```python
from build123d import *

# Parameters (mm, degrees)
F1_DEPTH = 5


with BuildPart() as f1:
    # F0 (on Top) → F1 (new body)
    with BuildSketch(Plane.XY):
        with BuildLine():
            ThreePointArc((3.1956666573, -6.9824714928), (2.7675285072, -8.5803048214), (1.5978333287, -9.75))
            Line((1.5978333287, -9.75), (4.793499986, -9.75))
            ThreePointArc((4.793499986, -9.75), (4.3653618359, -8.1521666713), (3.1956666573, -6.9824714928))
        make_face()
        with BuildLine():
            Line((-4.793499986, -9.75), (-1.5978333286, -9.75))
            ThreePointArc((-1.5978333286, -9.75), (-2.7675285072, -8.5803048214), (-3.1956666573, -6.9824714928))
            ThreePointArc((-3.1956666573, -6.9824714928), (-4.3653618359, -8.1521666713), (-4.793499986, -9.75))
        make_face()
        with BuildLine():
            ThreePointArc((3.1956666573, -6.9824714928), (4.3653618359, -8.1521666713), (4.793499986, -9.75))
            Line((4.793499986, -9.75), (12.3826613305, -9.75))
            Line((12.3826613305, -9.75), (17.9021666714, -9.75))
            ThreePointArc((17.9021666714, -9.75), (13.2777422874, 2.8582215277), (1.5978333286, 9.4863643814))
            Line((1.5978333286, 9.4863643814), (1.5978333287, -4.2149429855))
            ThreePointArc((1.5978333286, -4.2149429855), (2.7675285072, -5.3846381641), (3.1956666573, -6.9824714928))
        make_face()
        with BuildLine():
            Line((-17.9021666713, -9.75), (-4.793499986, -9.75))
            ThreePointArc((-4.793499986, -9.75), (-4.3653618359, -8.1521666713), (-3.1956666573, -6.9824714928))
            ThreePointArc((-3.1956666573, -6.9824714928), (-2.7675285072, -5.3846381641), (-1.5978333287, -4.2149429855))
            Line((-1.5978333286, -4.2149429855), (-1.5978333287, 9.4863643814))
            ThreePointArc((-1.5978333287, 9.4863643814), (-13.2777422874, 2.8582215277), (-17.9021666713, -9.75))
        make_face()
        with BuildLine():
            ThreePointArc((-1.5978333287, -4.2149429855), (0, -3.7868048355), (1.5978333286, -4.2149429855))
            Line((1.5978333287, -4.2149429855), (1.5978333286, 9.4863643814))
            ThreePointArc((1.5978333286, 9.4863643814), (0.8009617163, 9.6018935077), (0, 9.6844263783))
            ThreePointArc((0, 9.6844263783), (-0.8009617163, 9.6018935077), (-1.5978333287, 9.4863643814))
            Line((-1.5978333287, 9.4863643814), (-1.5978333286, -4.2149429855))
        make_face()
        with BuildLine():
            Line((-21.0978333287, -9.75), (-17.9021666713, -9.75))
            ThreePointArc((-17.9021666713, -9.75), (-13.2777422874, 2.8582215277), (-1.5978333287, 9.4863643814))
            Line((-1.5978333287, 9.4863643814), (-1.5978333287, 9.75))
            ThreePointArc((-1.5978333287, 9.75), (-15.3864155618, 4.0385822331), (-21.0978333286, -9.75))
        make_face()
        with BuildLine():
            ThreePointArc((0, 9.6844263783), (0.8009617163, 9.6018935077), (1.5978333286, 9.4863643814))
            Line((1.5978333286, 9.4863643814), (1.5978333286, 9.75))
            ThreePointArc((1.5978333286, 9.75), (0.798244177, 9.7335996979), (0, 9.6844263783))
        make_face()
        with BuildLine():
            Line((1.5978333286, 9.75), (1.5978333286, 9.4863643814))
            ThreePointArc((1.5978333286, 9.4863643814), (13.2777422874, 2.8582215277), (17.9021666714, -9.75))
            Line((17.9021666714, -9.75), (21.0978333287, -9.75))
            ThreePointArc((21.0978333287, -9.75), (15.3864155618, 4.0385822331), (1.5978333286, 9.75))
        make_face()
        with BuildLine():
            Line((-1.5978333287, 9.75), (-1.5978333287, 9.4863643814))
            ThreePointArc((-1.5978333287, 9.4863643814), (-0.8009617163, 9.6018935077), (0, 9.6844263783))
            ThreePointArc((0, 9.6844263783), (-0.798244177, 9.7335996979), (-1.5978333287, 9.75))
        make_face()
        with BuildLine():
            ThreePointArc((0, 9.6844263783), (0.798244177, 9.7335996979), (1.5978333286, 9.75))
            Line((1.5978333286, 9.75), (-1.5978333287, 9.75))
            ThreePointArc((-1.5978333287, 9.75), (-0.798244177, 9.7335996979), (0, 9.6844263783))
        make_face()
    extrude(amount=F1_DEPTH)


solid = f1.part
```
Geometry: final body of the model. Coordinates: model frame, mm. Coordinates: 2 decimals unless noted, no trailing zeros. Order: outer loops, then holes, each group sorted by start corner. A loop starts at its lowest first (then second) coordinate and runs counter-clockwise, first axis right, second up. Notation, with made-up numbers: (37, 17) - (49, 17) arc R25 cw to (49, 53) - close; hole circle Ø6 at (17, 68). An arc over 180 degrees is marked (long way). Return JSON: item names as keys, results as strings. Group by question number.
1. Cut plane B-B (y = -5.75). Output: boundary loops of the cut face in (x, z).
2. Material intervals for line 1 along Y through (x, z) = (0, 0.9); line 2 along X through (y, z) = (-4.75, 4.55); line 3 along X through (y, z) = (-5, 0.45), sorted ascending. Write a range as [from, to].
3. Cut plane C-C (x = 12.5). Output: boundary loops of the cut face in (y, z), plus the area to 3 significant figures.
4. Pin query (flat end, axial travel): pin 1 (2 mm diameter, centred on y = -2.5, z = 2, fed in from +X). Return the tip coordinate at first contact, or that it passes through.
5. Cut plane D-D (y = 1.5). Output: boundary loops of the cut face in (x, z).
6. Cut plane A-A (z = 1.9). Output: boundary loops of the cut face in (x, y), plus the area to 3 significant figures.
Resolved:
{
 "1": {"outline": "(-20.68, 0) - (-2.95, 0) - (-2.95, 5) - (-20.68, 5) - close; (2.95, 0) - (20.68, 0) - (20.68, 5) - (2.95, 5) - close"},
 "2": {"line 1": "y = [-3.79, 9.75]", "line 2": "x = [-20.45, -2.29], [2.29, 20.45]", "line 3": "x = [-20.51, -2.51], [2.51, 20.51]"},
 "3": {"outline": "(-9.75, 0) - (6.42, 0) - (6.42, 5) - (-9.75, 5) - close", "area": "80.8 mm²"},
 "4": {"pin 1": "stops at x = 20.07"},
 "5": {"outline": "(-17.53, 0) - (17.53, 0) - (17.53, 5) - (-17.53, 5) - close"},
 "6": {"outline": "(-21.1, -9.75) - (-1.6, -9.75) arc R3.2 cw (long way) to (1.6, -9.75) - (21.1, -9.75) arc R19.5 ccw to (1.6, 9.75) - (-1.6, 9.75) arc R19.5 ccw to start", "area": "628 mm²"}
}
